For this review, take the finished solid that the model builds, in its own axes (mm). Face numbers are marked on the shaded views. A direction names the side the tool comes from. Give positions to 0.01 mm unless a question says otherwise; leave off trailing zeros. Order: outer loops, then holes, each group sorted by start corner. A loop starts at its lowest first (then second) coordinate and runs counter-clockwise, first axis right, second up. Notation, with made-up numbers: M 6.25,-13.75 L 11.25,-13.75 A24 cw 11.25,-2.75 Z; hole C -34,82 d8. An arc over 180 degrees is marked long. Answer as CSV lines item,"result". Start each with the question number.
1. We need section C-C, the plane x = 140.5. Give the boundary of the cut face in (y, z).
2. We need section A-A, the plane x = 65. Give the boundary of the cut face in (y, z).
3. Machinability: for the marked faces 1 and 2, which of the approach directions +Z, -Z, +X, -X, +Y, -Y give a long, thin tool a straight path to every point of the face, cutting with its end or side? Answer none if there is none.
4. We need section B-B, the plane y = -14.5. Give the boundary of the cut face in (x, z), and give its area (3 significant figures).
5. For line 1 along Y through (x, z) = (-10, -0.3); line 2 along Y through (x, z) = (-10, -0.5); line 3 along Y through (x, z) = (132, -5.25), list the stretches that pass through material, from the lowest coordinate up.
6. Clearance check with flat-ended pins moving along their axes: P1, Ø2.5, axis at x = -10, y = -10, coming from the -Z side; P2, Ø8, axis at x = 117.5, z = -13.5, coming from the -Y side; P3, Ø10, axis at x = 64, y = -13, coming from the +Z side; P4, Ø3.5, axis at x = 10, y = 10, coming from the -Z side. State where each tip first meets the part, or that it passes through.
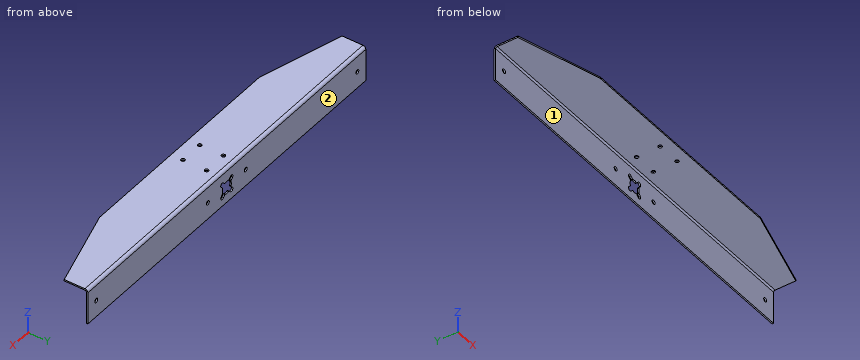
from build123d import *

# Parameters (mm, degrees)
SKETCH2_R                    = 1.6
BASE_FLANGE1_DEPTH           = 1.21412
EDGE_FLANGE1_STRIP_W         = 7.39648
EDGE_FLANGE1_STRIP_H         = 1.21412
EDGE_FLANGE1_STRIP_CUT_DEPTH = 330
EDGE_FLANGE1_DEPTH           = 330
CUT_EXTRUDE1_DEPTH           = 1.21412
SKETCH11_R                   = 1.75
CUT_EXTRUDE2_DEPTH           = 1.21412


# Sheet-metal steps are written as plain solids
with BuildPart() as part:
    # Sketch2 → Base-Flange1 (new body)
    with BuildSketch(Plane.XY):
        Polygon((-165, 0), (-165, 20), (165, 20), (165, 0), (95, -20), (-95, -20), align=None)
        with Locations((-10, 10)):
            Circle(SKETCH2_R, mode=Mode.SUBTRACT)
        with Locations((10, 10)):
            Circle(SKETCH2_R, mode=Mode.SUBTRACT)
        with Locations((10, -10)):
            Circle(SKETCH2_R, mode=Mode.SUBTRACT)
        with Locations((-10, -10)):
            Circle(SKETCH2_R, mode=Mode.SUBTRACT)
    extrude(amount=-BASE_FLANGE1_DEPTH)

    # Edge-Flange1 strip (across the edge) → Edge-Flange1 strip cut (cut)
    with BuildSketch(Plane(origin=(-165, 20, -1.21412), x_dir=(0, -1, 0), z_dir=(1, 0, 0))):
        with Locations((-1.21412, -0.60706)):
            Rectangle(EDGE_FLANGE1_STRIP_W, EDGE_FLANGE1_STRIP_H)
    extrude(amount=EDGE_FLANGE1_STRIP_CUT_DEPTH, mode=Mode.SUBTRACT)

    # Edge-Flange1 section (across the edge) → Edge-Flange1 (add)
    with BuildSketch(Plane(origin=(-165, 20, -1.21412), x_dir=(0, -1, 0), z_dir=(1, 0, 0))):
        with BuildLine():
            Line((0, 1.27), (0, 28.78588))
            Line((0, 28.78588), (1.21412, 28.78588))
            Line((1.21412, 28.78588), (1.21412, 1.27))
            ThreePointArc((1.21412, 1.27), (1.586094388, 0.371974388), (2.48412, 0))
            Line((2.48412, 0), (2.48412, -1.21412))
            ThreePointArc((2.48412, -1.21412), (0.727581903, -0.486538097), (0, 1.27))
        make_face()
    extrude(amount=EDGE_FLANGE1_DEPTH)

    # Sketch10 → Cut-Extrude1 (cut)
    with BuildSketch(Plane(origin=(0, 20, 0), x_dir=(1, 0, 0), z_dir=(0, 1, 0))):
        with BuildLine():
            Line((6.717514421, 21.028520687), (5.171899982, 19.482906248))
            ThreePointArc((5.171899982, 19.482906248), (4.968885146, 19.109755124), (5.001136207, 18.686179093))
            ThreePointArc((5.001136207, 18.686179093), (5.35, 16.78588), (5.001136207, 14.885580908))
            ThreePointArc((5.001136207, 14.885580908), (4.968885146, 14.462004877), (5.171899982, 14.088853753))
            Line((5.171899982, 14.088853753), (6.717514421, 12.543239313))
            ThreePointArc((6.717514421, 12.543239313), (6.717514421, 10.068365579), (4.242640687, 10.068365579))
            Line((4.242640687, 10.068365579), (2.697026248, 11.613980018))
            ThreePointArc((2.697026248, 11.613980018), (2.323875124, 11.816994854), (1.900299093, 11.784743793))
            ThreePointArc((1.900299093, 11.784743793), (0, 11.43588), (-1.900299092, 11.784743793))
            ThreePointArc((-1.900299092, 11.784743793), (-2.323875123, 11.816994854), (-2.697026247, 11.613980018))
            Line((-2.697026247, 11.613980018), (-4.242640687, 10.068365579))
            ThreePointArc((-4.242640687, 10.068365579), (-6.717514421, 10.068365579), (-6.717514421, 12.543239313))
            Line((-6.717514421, 12.543239313), (-5.171899982, 14.088853753))
            ThreePointArc((-5.171899982, 14.088853753), (-4.968885146, 14.462004877), (-5.001136207, 14.885580908))
            ThreePointArc((-5.001136207, 14.885580908), (-5.35, 16.78588), (-5.001136207, 18.686179093))
            ThreePointArc((-5.001136207, 18.686179093), (-4.968885146, 19.109755124), (-5.171899982, 19.482906248))
            Line((-5.171899982, 19.482906248), (-6.717514421, 21.028520687))
            ThreePointArc((-6.717514421, 21.028520687), (-6.717514421, 23.503394421), (-4.242640687, 23.503394421))
            Line((-4.242640687, 23.503394421), (-2.697026247, 21.957779982))
            ThreePointArc((-2.697026247, 21.957779982), (-2.323875123, 21.754765146), (-1.900299092, 21.787016207))
            ThreePointArc((-1.900299092, 21.787016207), (0, 22.13588), (1.900299093, 21.787016207))
            ThreePointArc((1.900299093, 21.787016207), (2.323875124, 21.754765146), (2.697026248, 21.957779982))
            Line((2.697026248, 21.957779982), (4.242640687, 23.503394421))
            ThreePointArc((4.242640687, 23.503394421), (6.717514421, 23.503394421), (6.717514421, 21.028520687))
        make_face()
    extrude(amount=-CUT_EXTRUDE1_DEPTH, mode=Mode.SUBTRACT)

    # Sketch11 → Cut-Extrude2 (cut)
    with BuildSketch(Plane(origin=(0, 20, 0), x_dir=(1, 0, 0), z_dir=(0, 1, 0))):
        with Locations(Location((-155, 15.78588, 0), (0, 0, 270))):
            Circle(SKETCH11_R)
        with Locations(Location((-22.5, 15.78588, 0), (0, 0, 270))):
            Circle(SKETCH11_R)
        with Locations(Location((22.5, 15.78588, 0), (0, 0, 270))):
            Circle(SKETCH11_R)
        with Locations(Location((155, 15.78588, 0), (0, 0, 270))):
            Circle(SKETCH11_R)
    extrude(amount=-CUT_EXTRUDE2_DEPTH, mode=Mode.SUBTRACT)


solid = part.part
Result set:
1,outline,"M -7,-1.21 L 17.52,-1.21 A1.27 cw 18.79,-2.48 L 18.79,-30 L 20,-30 L 20,-2.48 A2.48 ccw 17.52,0 L -7,0 Z"
2,outline,"M -20,-1.21 L 17.52,-1.21 A1.27 cw 18.79,-2.48 L 18.79,-30 L 20,-30 L 20,-2.48 A2.48 ccw 17.52,0 L -20,0 Z"
3,face 1,"-Z, +X, -X, -Y"
3,face 2,"+Z, -Z, +X, -X, +Y"
4,outline,"M -114.25,-1.21 L 114.25,-1.21 L 114.25,0 L -114.25,0 Z"
4,area,"277 mm2"
5,line 1,"-20 to -11.6, -8.4 to 8.4, 11.6 to 18.7"
5,line 2,"-20 to -11.6, -8.4 to 8.4, 11.6 to 19.01"
5,line 3,"18.79 to 20"
6,P1,"through"
6,P2,"y = 18.79"
6,P3,"z = 0"
6,P4,"z = -1.21"
